Part model, mm, in its own coordinate system. A direction names the side the tool comes from. Give positions to 0.01 mm unless a question says otherwise; leave off trailing zeros. Order: outer loops, then holes, each group sorted by start corner. A loop starts at its lowest first (then second) coordinate and runs counter-clockwise, first axis right, second up. Notation, with made-up numbers: M 7,-22 L 15,-22 A13 ccw 15,2 Z; hole C 63.5,86 d2. An arc over 180 degrees is marked long. Return JSON: item names as keys, results as strings.
from build123d import *

# Parameters (mm, degrees)
F0_W     = 25.4
F0_H     = 25.4
F1_DEPTH = 2.54
F3_DEPTH = 12.7
F4_W     = 2.540944
F4_H     = 3.556
F5_DEPTH = 12.7


with BuildPart() as f1:
    # F0 (on Top) → F1 (new body)
    with BuildSketch(Plane.XY):
        Rectangle(F0_W, F0_H)
    extrude(amount=-F1_DEPTH)

    # F2 (on Front) → F3 (join, symmetric)
    with BuildSketch(Plane.XZ):
        Polygon((-8.899515, -2.54), (-10.169515, -2.54), (-10.169515, -3.3528), (-11.44146, -4.192284), (-11.439515, -5.970282), (-8.899515, -5.969), align=None)
        Polygon((11.44146, -4.192284), (10.169515, -3.3528), (10.169515, -2.54), (8.899515, -2.54), (8.899515, -5.969), (11.439515, -5.970282), align=None)
    extrude(amount=F3_DEPTH, both=True)

    # F4 (on Right) → F5 (cut, symmetric)
    with BuildSketch(Plane.YZ):
        with Locations((11.429528, -4.318)):
            Rectangle(F4_W, F4_H)
    extrude(amount=F5_DEPTH, both=True, mode=Mode.SUBTRACT)


solid = f1.part
Q1. Band-saw the part on A-A (y = -10.25). Give the cut face in (x, z), then the cut area to 3 significant figures.
Established:
{"outline": "M -12.7,-2.54 L -10.17,-2.54 L -10.17,-3.35 L -11.44,-4.19 L -11.44,-5.97 L -8.9,-5.97 L -8.9,-2.54 L 8.9,-2.54 L 8.9,-5.97 L 11.44,-5.97 L 11.44,-4.19 L 10.17,-3.35 L 10.17,-2.54 L 12.7,-2.54 L 12.7,0 L -12.7,0 Z", "area": "78.8 mm²"}
Q2. Band-saw the part on C-C (x = 1.75). Give the cut face in (y, z), then the cut area to 3 significant figures.
Established:
{"outline": "M -12.7,-2.54 L 12.7,-2.54 L 12.7,0 L -12.7,0 Z", "area": "64.5 mm²"}
Q3. Pin check, flat tips, straight feed: pin 1 (3 mm diameter, centred on x = -5.5, y = 2.5, fed in from +Z); pin 2 (0.8 mm diameter, centred on x = -10.5, z = -4.5, fed in from +Y); pin 3 (1.7 mm diameter, centred on y = 4.5, z = -4.5, fed in from +X); pin 4 (4 mm diameter, centred on x = 0, y = -7.5, fed in from -Z). Stop position of each tip, or through.
Established:
{"pin 1": "stops at z = 0", "pin 2": "stops at y = 10.16", "pin 3": "stops at x = 11.44", "pin 4": "stops at z = -2.54"}
Q4. 3-axis set-ups, long thin cutter, end or side, ignore diameter. For faces 1 (the flat face through (10, 10.159, -5)), 2 (the flat face through (-10.8, -1.11, -3.77)), 3 (the flat face through (-8.9, -1, -4)): which of +Z, -Z, +X, -X, +Y, -Y reach the whole face in a straight line?
Established:
{"face 1": "-Z, +X, -X, +Y", "face 2": "-X, +Y, -Y", "face 3": "-Z, +Y, -Y"}
Q5. Two-plate mould, pull along Z, no slides. Class faces 4 (the flat face through (10.17, -1, -3)), 5 (the flat face through (0, 0, 0)), 6 (the flat face through (-10, 10.159, -5)): +Z half, -Z half, draft (parallel to the pull), parting line (faces both ways), or undercut.
Established:
{"face 4": "undercut", "face 5": "+Z half", "face 6": "draft"}
Q6. Probe line 1 along X through (y, z) = (7.25, -4.45); line 2 along Y through (x, z) = (9.5, -3.4); line 3 along Z through (x, y) = (-4.25, -10). List the from-to ranges inside material, lowest first.
Established:
{"line 1": "x = -11.44 to -8.9, 8.9 to 11.44", "line 2": "y = -12.7 to 10.16", "line 3": "z = -2.54 to 0"}
Q7. Band-saw the part on B-B (z = -4.7). Give the cut face in (x, y), then the cut area to 3 significant figures.
Established:
{"outline": "M -11.44,-12.7 L -8.9,-12.7 L -8.9,10.16 L -11.44,10.16 Z; M 8.9,-12.7 L 11.44,-12.7 L 11.44,10.16 L 8.9,10.16 Z", "area": "116 mm²"}
